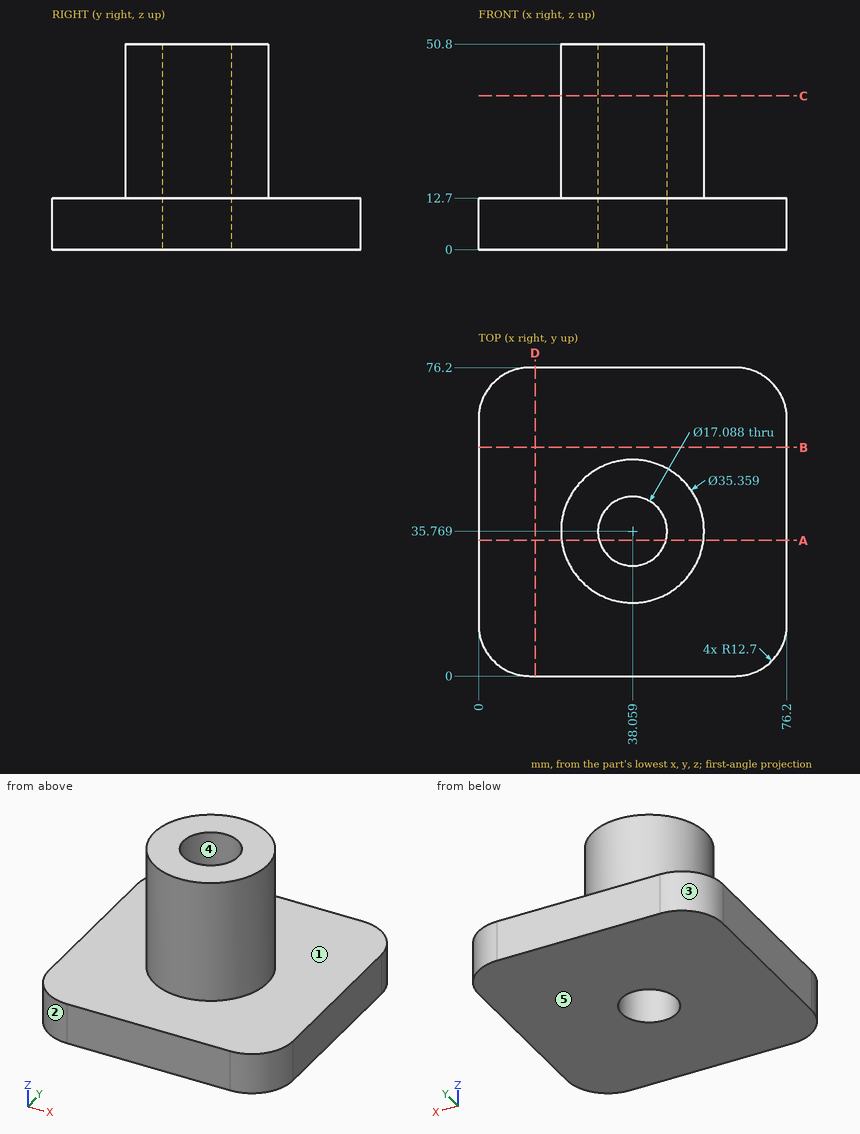
Study the drawing (mm; zero at the part's minimum x, y, z) and answer. A direction names the side the tool comes from. Coordinates: 2 decimals unless noted, no trailing zeros. Write each loop counter-clockwise with the first axis right and the second up, starting at its lowest first coordinate (ties: lowest second). Pieces come first, ordered by that corner, then holes. Notation, with made-up numbers: (-9, -26.75) - (5, -26.75) arc R20 ccw to (5, -7.75) - close; hole circle Ø8 at (50, 26.5). An arc over 180 degrees is marked (long way). One line per item, written item: value.
1) Consider line 1 along Z through (x, y) = (9.5, 60); line 2 along X through (y, z) = (12, 9); line 3 along Y through (x, z) = (31, 34) (1 decimal). Determine where each line is inside the solid, lowest interval first. Write a range as from..to.
Geometry check:
line 1: z = 0..12.7
line 2: x = 0.02..76.18
line 3: y = 19.6..31, 40.6..52
2) A tool of negligible diameter and unlimited length cuts with its end or side. For the marked faces 1 and 2, from which of +Z, -Z, +X, -X, +Y, -Y can it reach the whole face along a straight path? Write none if from no direction.
Geometry check:
face 1: +Z
face 2: +Z, -Z, -X, -Y
3) Find section A-A (y = 33.5). Give the vertices of the cut face in (x, z), and give its area (3 significant figures).
Geometry check:
outline: (0, 0) - (29.82, 0) - (29.82, 50.8) - (20.53, 50.8) - (20.53, 12.7) - (0, 12.7) - close; (46.3, 0) - (76.2, 0) - (76.2, 12.7) - (55.59, 12.7) - (55.59, 50.8) - (46.3, 50.8) - close
area: 1,470 mm2
4) Find section B-B (y = 56.5). Give the vertices of the cut face in (x, z).
Geometry check:
outline: (0, 0) - (76.2, 0) - (76.2, 12.7) - (0, 12.7) - close
5) Each of these flat-tipped pins is pushed along its axis until it touches: pin 1 Ø1 at (x, y) = (18.5, 38) entering from +Z; pin 2 Ø3 at (x, z) = (55.5, 41.5) entering from -Y (1 decimal); pin 3 Ø4 at (x, z) = (25.5, 41) entering from -Y. Where does it stop, or does it pass through?
Geometry check:
pin 1: stops at z = 12.7
pin 2: stops at y = 28.1
pin 3: stops at y = 21.59
6) For a pull along X with two mould halves and no side action, classify the marked faces 3, 4 and 5 as pulls with the +X half, pulls with the -X half, needs draft (parallel to the pull), parting line crosses it, or undercut.
Geometry check:
face 3: pulls with the -X half
face 4: undercut
face 5: needs draft
7) Find section C-C (z = 38). Give the vertices of the cut face in (x, y), and give its area (3 significant figures).
Geometry check:
outline: circle Ø35.36 at (38.06, 35.77); hole circle Ø17.09 at (38.06, 35.77)
area: 753 mm2
